from build123d import *

# Parameters (mm, degrees)
SKETCH1_W           = 165.1
SKETCH1_H           = 63.5
BOSS_EXTRUDE1_DEPTH = 3
CUT_EXTRUDE1_REACH  = 90.496
SKETCH6_R           = 1.5
SKETCH6_W           = 15
SKETCH6_H           = 10
CUT_EXTRUDE3_REACH  = 90.496
SKETCH8_R           = 2.38125
SKETCH9_R           = 2.0828
CUT_EXTRUDE5_DEPTH  = 5.08
SKETCH10_R          = 2.0828
CUT_EXTRUDE6_DEPTH  = 5.08


with BuildPart() as part:
    # Sketch1 → Boss-Extrude1 (new body)
    with BuildSketch(Plane(origin=(0, 0, 0), x_dir=(1, 0, 0), z_dir=(0, 1, 0))):
        Rectangle(SKETCH1_W, SKETCH1_H)
    extrude(amount=BOSS_EXTRUDE1_DEPTH)

    # Sketch6 → Cut-Extrude1 (cut, up to next)
    with BuildSketch(Plane.XZ, mode=Mode.PRIVATE) as cut_extrude1_sk1:
        with Locations(Location((-15.25, 15.25, 0), (0, 0, 270))):
            Circle(SKETCH6_R)
    cut_extrude1_tool1 = extrude(cut_extrude1_sk1.sketch, amount=-CUT_EXTRUDE1_REACH, mode=Mode.PRIVATE) & part.part
    # Sketch6 → Cut-Extrude1 (cut, up to next)
    with BuildSketch(Plane.XZ, mode=Mode.PRIVATE) as cut_extrude1_sk2:
        with Locations(Location((15.25, 15.25, 0), (0, 0, 270))):
            Circle(SKETCH6_R)
    cut_extrude1_tool2 = extrude(cut_extrude1_sk2.sketch, amount=-CUT_EXTRUDE1_REACH, mode=Mode.PRIVATE) & part.part
    # Sketch6 → Cut-Extrude1 (cut, up to next)
    with BuildSketch(Plane.XZ, mode=Mode.PRIVATE) as cut_extrude1_sk3:
        with Locations(Location((-15.25, -15.25, 0), (0, 0, 270))):
            Circle(SKETCH6_R)
    cut_extrude1_tool3 = extrude(cut_extrude1_sk3.sketch, amount=-CUT_EXTRUDE1_REACH, mode=Mode.PRIVATE) & part.part
    # Sketch6 → Cut-Extrude1 (cut, up to next)
    with BuildSketch(Plane.XZ, mode=Mode.PRIVATE) as cut_extrude1_sk4:
        with Locations(Location((15.25, -15.25, 0), (0, 0, 270))):
            Circle(SKETCH6_R)
    cut_extrude1_tool4 = extrude(cut_extrude1_sk4.sketch, amount=-CUT_EXTRUDE1_REACH, mode=Mode.PRIVATE) & part.part
    # Sketch6 → Cut-Extrude1 (cut, up to next)
    with BuildSketch(Plane.XZ, mode=Mode.PRIVATE) as cut_extrude1_sk5:
        with Locations((-43.3, 0.047)):
            Rectangle(SKETCH6_W, SKETCH6_H)
    cut_extrude1_tool5 = extrude(cut_extrude1_sk5.sketch, amount=-CUT_EXTRUDE1_REACH, mode=Mode.PRIVATE) & part.part
    add(cut_extrude1_tool1.solids().sort_by_distance((-15.25, 0, 15.25))[0], mode=Mode.SUBTRACT)
    add(cut_extrude1_tool2.solids().sort_by_distance((15.25, 0, 15.25))[0], mode=Mode.SUBTRACT)
    add(cut_extrude1_tool3.solids().sort_by_distance((-15.25, 0, -15.25))[0], mode=Mode.SUBTRACT)
    add(cut_extrude1_tool4.solids().sort_by_distance((15.25, 0, -15.25))[0], mode=Mode.SUBTRACT)
    add(cut_extrude1_tool5.solids().sort_by_distance((-43.3, 0, 0.047))[0], mode=Mode.SUBTRACT)

    # Sketch8 → Cut-Extrude3 (cut, up to next)
    with BuildSketch(Plane(origin=(0, 3, 0), x_dir=(1, 0, 0), z_dir=(0, 1, 0)), mode=Mode.PRIVATE) as cut_extrude3_sk1:
        with Locations(Location((-63.5, -12.7, 0), (0, 0, 270))):
            Circle(SKETCH8_R)
    cut_extrude3_tool1 = extrude(cut_extrude3_sk1.sketch, amount=-CUT_EXTRUDE3_REACH, mode=Mode.PRIVATE) & part.part
    # Sketch8 → Cut-Extrude3 (cut, up to next)
    with BuildSketch(Plane(origin=(0, 3, 0), x_dir=(1, 0, 0), z_dir=(0, 1, 0)), mode=Mode.PRIVATE) as cut_extrude3_sk2:
        with Locations(Location((-63.5, 12.7, 0), (0, 0, 270))):
            Circle(SKETCH8_R)
    cut_extrude3_tool2 = extrude(cut_extrude3_sk2.sketch, amount=-CUT_EXTRUDE3_REACH, mode=Mode.PRIVATE) & part.part
    # Sketch8 → Cut-Extrude3 (cut, up to next)
    with BuildSketch(Plane(origin=(0, 3, 0), x_dir=(1, 0, 0), z_dir=(0, 1, 0)), mode=Mode.PRIVATE) as cut_extrude3_sk3:
        with Locations(Location((63.5, 12.7, 0), (0, 0, 270))):
            Circle(SKETCH8_R)
    cut_extrude3_tool3 = extrude(cut_extrude3_sk3.sketch, amount=-CUT_EXTRUDE3_REACH, mode=Mode.PRIVATE) & part.part
    # Sketch8 → Cut-Extrude3 (cut, up to next)
    with BuildSketch(Plane(origin=(0, 3, 0), x_dir=(1, 0, 0), z_dir=(0, 1, 0)), mode=Mode.PRIVATE) as cut_extrude3_sk4:
        with Locations(Location((63.5, -12.7, 0), (0, 0, 270))):
            Circle(SKETCH8_R)
    cut_extrude3_tool4 = extrude(cut_extrude3_sk4.sketch, amount=-CUT_EXTRUDE3_REACH, mode=Mode.PRIVATE) & part.part
    add(cut_extrude3_tool1.solids().sort_by_distance((-63.5, 3, 12.7))[0], mode=Mode.SUBTRACT)
    add(cut_extrude3_tool2.solids().sort_by_distance((-63.5, 3, -12.7))[0], mode=Mode.SUBTRACT)
    add(cut_extrude3_tool3.solids().sort_by_distance((63.5, 3, -12.7))[0], mode=Mode.SUBTRACT)
    add(cut_extrude3_tool4.solids().sort_by_distance((63.5, 3, 12.7))[0], mode=Mode.SUBTRACT)

    # Sketch9 → Cut-Extrude5 (cut)
    with BuildSketch(Plane(origin=(0, 3, 0), x_dir=(1, 0, 0), z_dir=(0, 1, 0))):
        with Locations(Location((-75.692, 0, 0), (0, 0, 270))):
            Circle(SKETCH9_R)
        with Locations(Location((75.692, 0, 0), (0, 0, 270))):
            Circle(SKETCH9_R)
    extrude(amount=-CUT_EXTRUDE5_DEPTH, mode=Mode.SUBTRACT)

    # Sketch10 → Cut-Extrude6 (cut)
    with BuildSketch(Plane(origin=(0, 3, 0), x_dir=(1, 0, 0), z_dir=(0, 1, 0))):
        with Locations(Location((0, -24.892, 0), (0, 0, 270))):
            Circle(SKETCH10_R)
        with Locations(Location((0, 24.892, 0), (0, 0, 270))):
            Circle(SKETCH10_R)
    extrude(amount=-CUT_EXTRUDE6_DEPTH, mode=Mode.SUBTRACT)


solid = part.part
For this review, take the finished solid that the model builds, in its own axes (mm). A direction names the side the tool comes from. Give positions to 0.01 mm unless a question says otherwise; leave off trailing zeros. Loops run counter-clockwise (first coordinate to the right, second up) from the corner with the lowest first, then second, coordinate; pieces in that order, holes last. Notation, with made-up numbers: M 60.5,-7 L 113.5,-7 A22 cw 113.5,5 Z; hole C -27,-22 d7. An arc over 180 degrees is marked long. Put each result on its own line as item: value. Start each with the question number.
(1) Add section D-D, the plane x = 15.25. Write out the cut boundary in (y, z).
(2) Wall thickness on L1, parallel to X at y = 1.55, z = 13; L2, parallel to X at y = 1.2, z = 0; L3, parallel to Z at x = -38, y = 2.3: over which ranges is each line inside the solid? List them lowest first.
(3) For pin 1 (2.5 mm diameter, centred on x = -15.25, z = 15.25, fed in from +Y); pin 2 (6.5 mm diameter, centred on x = 75.692, z = 0, fed in from +Y), all flat-tipped, find the tip position at first contact; note any pin that passes through.
(4) The part is to be moulded in two halves that separate along Z. For faces 3 (the cylindrical face through (-65.825, 1.521, 12.184)), 4 (the flat face through (-1, 1, -31.75)), 5 (the flat face through (-1, 0, 0)), say which applies: +Z half, -Z half, draft (parallel to the pull), parting line (faces both ways), or undercut.
(5) Add section C-C, the plane z = 25.5. Write out the cut boundary in (x, y), then the cut area to 3 significant figures.
(6) Add section A-A, the plane x = -63.5. Write out the cut boundary in (y, z), then the cut area to 3 significant figures.
(7) Machinability: for faces 1 (the flat face through (-82.55, 1, 0)), 2 (the flat face through (-50.8, 1, 0)), which of the approach directions +Z, -Z, +X, -X, +Y, -Y give a long, thin tool a straight path to every point of the face, cutting with its end or side? Answer none if there is none.
(8) Add section B-B, the plane y = 2.15. Give the number of separate pieces and of enclosed holes in the cut face, then the cut area to 3 significant figures.
Result:
1. outline: M 0,-31.75 L 3,-31.75 L 3,-16.75 L 0,-16.75 Z; M 0,-13.75 L 3,-13.75 L 3,13.75 L 0,13.75 Z; M 0,16.75 L 3,16.75 L 3,31.75 L 0,31.75 Z
2. L1: x = -82.55 to -65.86, -61.14 to 61.14, 65.86 to 82.55
2. L2: x = -82.55 to -77.77, -73.61 to -50.8, -35.8 to 73.61, 77.77 to 82.55
2. L3: z = -31.75 to -4.95, 5.05 to 31.75
3. pin 1: passes through
3. pin 2: stops at y = 3
4. face 3: undercut
4. face 4: -Z half
4. face 5: draft
5. outline: M -82.55,0 L -1.99,0 L -1.99,3 L -82.55,3 Z; M 1.99,0 L 82.55,0 L 82.55,3 L 1.99,3 Z
5. area: 483 mm^2
6. outline: M 0,-31.75 L 3,-31.75 L 3,-15.08 L 0,-15.08 Z; M 0,-10.32 L 3,-10.32 L 3,10.32 L 0,10.32 Z; M 0,15.08 L 3,15.08 L 3,31.75 L 0,31.75 Z
6. area: 162 mm^2
7. face 1: +Z, -Z, -X, +Y, -Y
7. face 2: +Y, -Y
8. separate pieces: 1
8. enclosed holes: 13
8. area: 10,200 mm^2
